Design review of the part shown in the three views and the two pictorial views. Dimensions are in mm from the part's minimum x, y and z. A direction names the side the tool comes from. Coordinates: 2 decimals unless noted, no trailing zeros. Order: outer loops, then holes, each group sorted by start corner. A loop starts at its lowest first (then second) coordinate and runs counter-clockwise, first axis right, second up. Notation, with made-up numbers: (67, 35.5) - (108, 35.5) arc R16 cw to (108, 39.5) - close; hole circle Ø2 at (45.25, 41). An arc over 180 degrees is marked (long way). One line per item, written item: value. Start each with the question number.
(1) To check wall thickness, follow line 1 along Y through (x, z) = (15.25, 10.5); line 2 along X through (y, z) = (11.25, 3). State the ranges of each line that lie inside material, in increasing order.
(2) Consider section B-B on x = 3.5. Write out the cut boundary in (y, z).
(3) For the marked faces 1, 2, 3 and 4, list the 3-axis set-ups (+Z, -Z, +X, -X, +Y, -Y) from which the entire face can be reached by the end or side of a thin tool; tool diameter is ignored.
(4) Consider section A-A on z = 31.5. Write out the cut boundary in (x, y), then the cut area to 3 significant figures.
(5) Clearance check with flat-ended pins moving along their axes: pin 1 (1.2 mm diameter, centred on x = 14.5, z = 12, fed in from -Y); pin 2 (3 mm diameter, centred on x = 3, z = 20, fed in from +Y); pin 3 (2 mm diameter, centred on y = 2, z = 21, fed in from +X); pin 4 (4 mm diameter, centred on x = 2.5, y = 3, fed in from -Z). State where each tip first meets the part, or that it passes through.
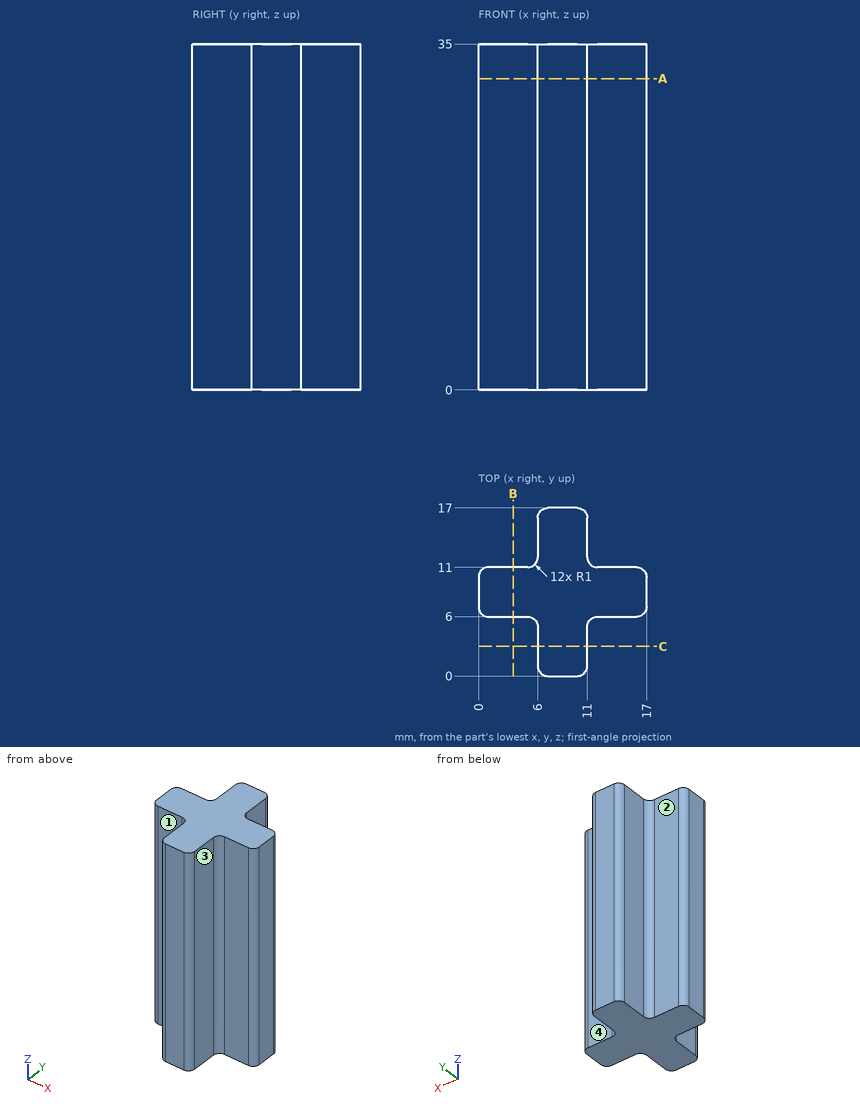
Geometry check:
1. line 1: y = 6 to 11
1. line 2: x = 5.66 to 11.34
2. outline: (6, 0) - (11, 0) - (11, 35) - (6, 35) - close
3. face 1: +Z, -Z, -X, -Y
3. face 2: +Z, -Z, -X, +Y
3. face 3: +Z, -Z, +X, -Y
3. face 4: +Z, -Z, +X, +Y
4. outline: (0, 7) arc R1 ccw to (1, 6) - (5, 6) arc R1 cw to (6, 5) - (6, 1) arc R1 ccw to (7, 0) - (10, 0) arc R1 ccw to (11, 1) - (11, 5) arc R1 cw to (12, 6) - (16, 6) arc R1 ccw to (17, 7) - (17, 10) arc R1 ccw to (16, 11) - (12, 11) arc R1 cw to (11, 12) - (11, 16) arc R1 ccw to (10, 17) - (7, 17) arc R1 ccw to (6, 16) - (6, 12) arc R1 cw to (5, 11) - (1, 11) arc R1 ccw to (0, 10) - close
4. area: 144 mm^2
5. pin 1: stops at y = 6
5. pin 2: stops at y = 11
5. pin 3: stops at x = 11
5. pin 4: passes through
